from build123d import *

# Parameters (mm, degrees)
BOSS_EXTRUDE1_DEPTH      = 30
BOSS_EXTRUDE1_DEPTH_BACK = 30
CHAMFER1_SIZE            = 20
FILLET1_R                = 15
FILLET2_R                = 5


with BuildPart() as part:
    # Sketch2 → Boss-Extrude1 (new body, two sides)
    with BuildSketch(Plane.XY) as boss_extrude1_sk:
        Polygon((-133.5, 85.338455572), (-88.5, 85.338455572), (-88.5, 0), (88.5, 0), (88.5, 164), (138.5, 164), (138.5, -57.5), (88.5, -57.5), (88.5, -50), (-83.5, -50), (-83.5, -57.5), (-133.5, -57.5), align=None)
    extrude(amount=BOSS_EXTRUDE1_DEPTH)
    extrude(boss_extrude1_sk.sketch, amount=-BOSS_EXTRUDE1_DEPTH_BACK)

    # Chamfer1
    chamfer1_edges = [part.edges().sort_by_distance(p)[0] for p in [
        (-133.5, 85.338455572, 0),
        (138.5, 164, 0),
        (138.5, -57.5, 0),
        (-133.5, -57.5, 0),
    ]]
    chamfer(chamfer1_edges, length=CHAMFER1_SIZE)

    # Fillet1
    fillet1_edges = [part.edges().sort_by_distance(p)[0] for p in [
        (-88.5, 0, 0),
        (88.5, 0, 0),
    ]]
    fillet(fillet1_edges, radius=FILLET1_R)

    # Fillet2
    fillet2_edges = [part.edges().sort_by_distance(p)[0] for p in [
        (-88.5, 85.338455572, 0),
        (88.5, 164, 0),
        (88.5, -50, 0),
        (-83.5, -50, 0),
        (-133.5, 65.338455572, 0),
        (-133.5, -37.5, 0),
        (138.5, 144, 0),
        (138.5, -37.5, 0),
        (118.5, 164, 0),
        (-113.5, 85.338455572, 0),
    ]]
    fillet(fillet2_edges, radius=FILLET2_R)


solid = part.part
Verification items for the finished model (mm, model axes). A direction names the side the tool comes from. Round coordinates to 2 decimals unless told otherwise and drop trailing zeros. Loops run counter-clockwise (first coordinate to the right, second up) from the corner with the lowest first, then second, coordinate; pieces in that order, holes last. Notation, with made-up numbers: (74, 29.5) - (111, 29.5) arc R10 ccw to (111, 47.5) - close; hole circle Ø5 at (-34, 84.25). An arc over 180 degrees is marked (long way). Answer in a Markdown table with one row per item. Add a question column.
Q1. Tool access check on faces 1 (the face through (-103, 85.338, 0)), 2 (the face through (-84.22, 4.51, -0.42)), 3 (the face through (128.4, 154.1, 0.4)), 4 (the face through (4, -50, 0)). Record the directions out of +Z, -Z, +X, -X, +Y, -Y that give a thin tool (end or side, any length) a straight path to the whole face; none if there is none.
Q2. Section check C-C on x = -104.5. Enter the section's corners in (y, z).
Q3. Material ranges on line 1 (X direction, y = 52, z = -8); line 2 (Y direction, x = -26, z = -7.5); line 3 (X direction, y = 124.5, z = -17.5), recorded low to high.
Q4. Section check A-A on y = 19. Enter the section's corners in (x, z), plus the area to 3 significant figures.
Q5. Section check B-B on z = -16. Enter the section's corners in (x, y).
Q6. Gauge pin test, flat ends, axial feed: pin 1 (18 mm diameter, centred on x = -27, z = -14.5, fed in from -Y); pin 2 (1.3 mm diameter, centred on y = -55.5, z = -10, fed in from +X); pin 3 (19.5 mm diameter, centred on x = -100.5, z = 10.5, fed in from +Y). Record the tip position at first contact, or that the pin passes through.
Q7. Section check D-D on y = 99.5. Enter the section's corners in (x, z), plus the area to 3 significant figures.
Found:
| question | item | result |
|---|---|---|
| 1 | face 1 | +Z, -Z, -X, +Y |
| 1 | face 2 | +Z, -Z, +Y |
| 1 | face 3 | +Z, -Z, +X, +Y |
| 1 | face 4 | +Z, -Z, -Y |
| 2 | outline | (-57.5, -30) - (85.34, -30) - (85.34, 30) - (-57.5, 30) - close |
| 3 | line 1 | x = -133.5 to -88.5, 88.5 to 138.5 |
| 3 | line 2 | y = -50 to 0 |
| 3 | line 3 | x = 88.5 to 138.5 |
| 4 | outline | (-133.5, -30) - (-88.5, -30) - (-88.5, 30) - (-133.5, 30) - close; (88.5, -30) - (138.5, -30) - (138.5, 30) - (88.5, 30) - close |
| 4 | area | 5,700 mm² |
| 5 | outline | (-133.5, -35.43) arc R5 ccw to (-132.04, -38.96) - (-113.5, -57.5) - (-83.5, -57.5) - (-83.5, -55) arc R5 cw to (-78.5, -50) - (83.5, -50) arc R5 cw to (88.5, -55) - (88.5, -57.5) - (118.5, -57.5) - (137.04, -38.96) arc R5 ccw to (138.5, -35.43) - (138.5, 141.93) arc R5 ccw to (137.04, 145.46) - (119.96, 162.54) arc R5 ccw to (116.43, 164) - (93.5, 164) arc R5 ccw to (88.5, 159) - (88.5, 15) arc R15 cw to (73.5, 0) - (-73.5, 0) arc R15 cw to (-88.5, 15) - (-88.5, 80.34) arc R5 ccw to (-93.5, 85.34) - (-111.43, 85.34) arc R5 ccw to (-114.96, 83.87) - (-132.04, 66.8) arc R5 ccw to (-133.5, 63.27) - close |
| 6 | pin 1 | stops at y = -50 |
| 6 | pin 2 | stops at x = 121.15 |
| 6 | pin 3 | stops at y = 85.34 |
| 7 | outline | (88.5, -30) - (138.5, -30) - (138.5, 30) - (88.5, 30) - close |
| 7 | area | 3,000 mm² |
